Geometry: final body of the model. Coordinates: model frame, mm. A direction names the side the tool comes from. Round coordinates to 2 decimals unless told otherwise and drop trailing zeros. Order: outer loops, then holes, each group sorted by start corner. A loop starts at its lowest first (then second) coordinate and runs counter-clockwise, first axis right, second up. Notation, with made-up numbers: M 67,-36.75 L 83,-36.75 A26 ccw 83,-14.75 Z; hole C 40,19 d10. An arc over 180 degrees is marked long. Return JSON: item names as keys, results as strings. Group by question number.
Q1. Cut plane C-C on x = -16.5. Output: boundary loops of the cut face in (y, z).
Q2. Cut plane D-D on x = -50.5. Output: boundary loops of the cut face in (y, z).
Q3. Mould query, pull axis Y, two halves, no side actions, for faces 6 (the face through (-94.86, 98.73, 98.38)), 7 (the face through (-105, 48, -48)), 8 (the face through (-9.86, 1.139, -93.676)). Classes: released by +Y, released by -Y, zero draft, split by the parting line, or undercut.
Q4. Ray query, probe 1 along X at (y, z) = (91, 20); probe 2 along Z at (x, y) = (-91, -80); probe 3 along Z at (x, y) = (-14.75, 0). Return the intervals inside material, ascending.
Q5. Access query for faces 1 (the face through (-95, -1, 105)), 2 (the face through (-9.86, -93.676, -1.139)), 3 (the face through (-85, 25, -48)), 4 (the face through (-95.14, -88.676, -78.861)), 5 (the face through (-95, -105, -1)). Directions: +Z, -Z, +X, -X, +Y, -Y. A direction counts if a zero-diameter tool reaches every point of the face in a straight line with its end or side. Return the directions, or none.
Q6. Contact query for flat-ended pins moving along their axis: pin 1 (16 mm diameter, centred on x = -97.5, y = -37, fed in from -Z); pin 2 (10 mm diameter, centred on y = -73.5, z = -12.5, fed in from -X); pin 3 (3 mm diameter, centred on x = -37.5, z = 48.5, fed in from -Y). Output: stop coordinate, or through.
Q7. Cut plane A-A on y = -80. Output: boundary loops of the cut face in (x, z).
```python
from build123d import *

# Parameters (mm, degrees)
SKETCH_2_R               = 8.75
CUT_EXTRUDE_1_DEPTH      = 20
PATTERN_CIRCULAR_1_COUNT = 4
SKETCH_3_W               = 210
SKETCH_3_H               = 210
SKETCH_3_R               = 35
EXTRUDE_1_DEPTH          = 20
SKETCH_4_R               = 8.75
CUT_EXTRUDE_2_DEPTH      = 20
FILLET_1_R               = 22
PATTERN_CIRCULAR_5_COUNT = 4
CHAMFER_1_SIZE           = 3.2875
FILLET_2_R               = 3


with BuildPart() as part:
    # Эскиз1 → Повернуть1 (revolve)
    with BuildSketch(Plane.XY):
        Polygon((0, 52.5), (0, 110), (-20, 110), (-20, 65), (-85, 50), (-85, 105), (-105, 105), (-105, 62.5), (-130, 62.5), (-130, 28.7125), (-113, 28.7125), (-113, 35), (-105, 35), (-105, 25), align=None)
    revolve(axis=Axis((0, 0, 0), (-1, 0, 0)))

    # Эскиз2 → Вырез-Вытянуть1 (cut)
    with BuildSketch(Plane(origin=(0, 0, 0), x_dir=(0, 0, -1), z_dir=(1, 0, 0))):
        with Locations((0, 85)):
            Circle(SKETCH_2_R)
    cut_extrude_1 = extrude(amount=-CUT_EXTRUDE_1_DEPTH, mode=Mode.SUBTRACT)

    # Круговой массив1: Вырез-Вытянуть1 ×4 about axis
    pattern_circular_1_axis = Axis((0, 0, 0), (1, 0, 0))
    for i in range(1, PATTERN_CIRCULAR_1_COUNT):
        add(cut_extrude_1.rotate(pattern_circular_1_axis, i * 360 / PATTERN_CIRCULAR_1_COUNT), mode=Mode.SUBTRACT)

    # Эскиз3 → Бобышка-Вытянуть1 (add)
    with BuildSketch(Plane.ZY.offset(105)):
        Rectangle(SKETCH_3_W, SKETCH_3_H)
        Circle(SKETCH_3_R, mode=Mode.SUBTRACT)
    extrude(amount=-EXTRUDE_1_DEPTH)

    # Эскиз4 → Вырез-Вытянуть2 (cut)
    with BuildSketch(Plane.ZY.offset(105)):
        with Locations((80, 80)):
            Circle(SKETCH_4_R)
    cut_extrude_2 = extrude(amount=-CUT_EXTRUDE_2_DEPTH, mode=Mode.SUBTRACT)

    # Скругление1
    fillet_1_edges = [part.edges().sort_by_distance(p)[0] for p in [
        (-95, 105, 105),
        (-95, -105, 105),
        (-95, -105, -105),
        (-95, 105, -105),
    ]]
    fillet(fillet_1_edges, radius=FILLET_1_R)

    # Круговой массив5: Вырез-Вытянуть2 ×4 about axis
    pattern_circular_5_axis = Axis((0, 0, 0), (1, 0, 0))
    for i in range(1, PATTERN_CIRCULAR_5_COUNT):
        add(cut_extrude_2.rotate(pattern_circular_5_axis, i * 360 / PATTERN_CIRCULAR_5_COUNT), mode=Mode.SUBTRACT)

    # Фаска1
    chamfer_1_edges = [part.edges().sort_by_distance(p)[0] for p in [
        (-130, -28.7125, 0),
    ]]
    chamfer(chamfer_1_edges, length=CHAMFER_1_SIZE)

    # Скругление2
    fillet_2_edges = [part.edges().sort_by_distance(p)[0] for p in [
        (-20, -65, 0),
        (-85, -50, 0),
    ]]
    fillet(fillet_2_edges, radius=FILLET_2_R)


solid = part.part
```
Result sheet:
{
 "1": {"outline": "C 0,0 d220; hole C -85,0 d17.5; hole C 0,0 d96.36; hole C 0,-85 d17.5; hole C 0,85 d17.5; hole C 85,0 d17.5"},
 "2": {"outline": "C 0,0 d115.92; hole C 0,0 d78.55"},
 "3": {"face 6": "released by +Y", "face 7": "zero draft", "face 8": "undercut"},
 "4": {"probe 1": "x = -105 to -85, -20 to 0", "probe 2": "z = -105 to -88.75, -71.25 to 71.25, 88.75 to 105", "probe 3": "z = -110 to -93.75, -76.25 to -48.64, 48.64 to 76.25, 93.75 to 110"},
 "5": {"face 1": "+Z, -X, +Y, -Y", "face 2": "+X", "face 3": "none", "face 4": "-X", "face 5": "+Z, -Z, -X, -Y"},
 "6": {"pin 1": "stops at z = -105", "pin 2": "stops at x = -105", "pin 3": "stops at y = -38.9"},
 "7": {"outline": "M -105,-105 L -85,-105 L -85,-88.75 L -105,-88.75 Z; M -105,-71.25 L -85,-71.25 L -85,71.25 L -105,71.25 Z; M -105,88.75 L -85,88.75 L -85,105 L -105,105 Z; M -20,-75.5 L 0,-75.5 L 0,-7.18 L -20,-7.18 Z; M -20,7.18 L 0,7.18 L 0,75.5 L -20,75.5 Z"}
}
